from build123d import *

# Parameters (mm, degrees)
SKETCH1_W               = 60
SKETCH1_H               = 160
BOSS_EXTRUDE1_DEPTH     = 3.175
M4_5_THROUGH_DEPTH      = 6.35
M4_5_THROUGH_DEPTH_BACK = 3.175
SKETCH3_R               = 2.75
SKETCH3_R_2             = 2.25
SKETCH4_R               = 1.5
M3_DRILL_DEPTH          = 8
SKETCH5_R               = 2.25
M4_THROUGH_DEPTH        = 6.35
SKETCH6_R               = 2.5
M5_DRILL_DEPTH          = 6.35
SKETCH7_R               = 2.75
M5_THROUGH_DEPTH        = 6.35
SKETCH8_W               = 60
SKETCH8_H               = 30.2375
CUT_EXTRUDE3_DEPTH      = 6.35


with BuildPart() as part:
    # Sketch1 → Boss-Extrude1 (new, symmetric)
    with BuildSketch(Plane(origin=(0, 0, 0), x_dir=(1, 0, 0), z_dir=(0, 1, 0))):
        Rectangle(SKETCH1_W, SKETCH1_H)
    extrude(amount=BOSS_EXTRUDE1_DEPTH, both=True)

    # Sketch3 → M4/5_through (cut, two sides: drawn at the far end of the back side and taken through both)
    with BuildSketch(Plane(origin=(0, 0, 0), x_dir=(1, 0, 0), z_dir=(0, 1, 0)).offset(-M4_5_THROUGH_DEPTH_BACK)):
        with Locations(Location((20, 75.2375, 0), (0, 0, 270))):
            Circle(SKETCH3_R)
        with Locations(Location((20, 50.2375, 0), (0, 0, 270))):
            Circle(SKETCH3_R_2)
        with Locations(Location((-20, 50.2375, 0), (0, 0, 270))):
            Circle(SKETCH3_R_2)
        with Locations(Location((-20, 75.2375, 0), (0, 0, 270))):
            Circle(SKETCH3_R)
        with Locations(Location((0, 75.2375, 0), (0, 0, 270))):
            Circle(SKETCH3_R)
        with Locations(Location((0, 50.2375, 0), (0, 0, 270))):
            Circle(SKETCH3_R_2)
        with Locations(Location((20, -44.7625, 0), (0, 0, 270))):
            Circle(SKETCH3_R_2)
        with Locations(Location((-20, -44.7625, 0), (0, 0, 270))):
            Circle(SKETCH3_R_2)
        with Locations(Location((0, -44.7625, 0), (0, 0, 270))):
            Circle(SKETCH3_R_2)
    extrude(amount=M4_5_THROUGH_DEPTH + M4_5_THROUGH_DEPTH_BACK, mode=Mode.SUBTRACT)

    # Sketch4 → M3_DRILL (cut)
    with BuildSketch(Plane(origin=(0, 0, -80), x_dir=(-1, 0, 0), z_dir=(0, 0, -1))):
        with Locations((-12, 0)):
            Circle(SKETCH4_R)
        with Locations(Location((12, 0, 0), (0, 0, 180))):
            Circle(SKETCH4_R)
    extrude(amount=-M3_DRILL_DEPTH, mode=Mode.SUBTRACT)

    # Sketch5 → M4_through (cut)
    with BuildSketch(Plane(origin=(0, 3.175, 0), x_dir=(1, 0, 0), z_dir=(0, 1, 0))):
        with Locations(Location((-25.2375, -27.6625, 0), (0, 0, 270))):
            Circle(SKETCH5_R)
        with Locations(Location((25.2375, -27.6625, 0), (0, 0, 270))):
            Circle(SKETCH5_R)
        with Locations(Location((25.2375, 33.1375, 0), (0, 0, 270))):
            Circle(SKETCH5_R)
        with Locations(Location((-25.2375, 33.1375, 0), (0, 0, 270))):
            Circle(SKETCH5_R)
    extrude(amount=-M4_THROUGH_DEPTH, mode=Mode.SUBTRACT)

    # Sketch6 → M5_DRILL (cut)
    with BuildSketch(Plane(origin=(0, 3.175, 0), x_dir=(1, 0, 0), z_dir=(0, 1, 0))):
        with Locations(Location((0, 30, 0), (0, 0, 270))):
            Circle(SKETCH6_R)
        with Locations(Location((9.53, 30, 0), (0, 0, 270))):
            Circle(SKETCH6_R)
        with Locations(Location((-9.53, 30, 0), (0, 0, 270))):
            Circle(SKETCH6_R)
    extrude(amount=-M5_DRILL_DEPTH, mode=Mode.SUBTRACT)

    # Sketch7 → M5_through (cut)
    with BuildSketch(Plane(origin=(0, 3.175, 0), x_dir=(1, 0, 0), z_dir=(0, 1, 0))):
        with Locations(Location((0, 10, 0), (0, 0, 270))):
            Circle(SKETCH7_R)
        with Locations(Location((0, -15, 0), (0, 0, 270))):
            Circle(SKETCH7_R)
        with Locations(Location((9.53, 10, 0), (0, 0, 270))):
            Circle(SKETCH7_R)
        with Locations(Location((9.53, -15, 0), (0, 0, 270))):
            Circle(SKETCH7_R)
        with Locations(Location((-9.53, 10, 0), (0, 0, 270))):
            Circle(SKETCH7_R)
        with Locations(Location((-9.53, -15, 0), (0, 0, 270))):
            Circle(SKETCH7_R)
    extrude(amount=-M5_THROUGH_DEPTH, mode=Mode.SUBTRACT)

    # Sketch8 → Cut-Extrude3 (cut)
    with BuildSketch(Plane(origin=(0, 3.175, 0), x_dir=(1, 0, 0), z_dir=(0, 1, 0))):
        with Locations((0, -64.88125)):
            Rectangle(SKETCH8_W, SKETCH8_H)
    extrude(amount=-CUT_EXTRUDE3_DEPTH, mode=Mode.SUBTRACT)


solid = part.part
Source: CAD feature listing. Evaluate the final solid. Frame: model axes, mm. A direction names the side the tool comes from. Coordinates: 2 decimals unless noted, no trailing zeros. Loops run counter-clockwise (first coordinate to the right, second up) from the corner with the lowest first, then second, coordinate; pieces in that order, holes last. Notation, with made-up numbers: (-23.75, 24.25) - (-17.75, 24.25) arc R24 ccw to (-17.75, 57.25) - close; hole circle Ø7 at (-34, -12.5). An arc over 180 degrees is marked (long way). One line per item, written item: value. Start each with the question number.
1. Set-up query: faces 4 (the cylindrical face through (0.099, -0.044, 42.515)), 5 (the cylindrical face through (13.5, 0.07, -76.06)). Return all of +Z, -Z, +X, -X, +Y, -Y with unobstructed straight access to the full face (end or side cutting, diameter ignored); none if empty.
2. Ray query, L1, parallel to Z at x = 20, y = -1.25; L2, parallel to Y at x = 12, z = -73.75 (3 decimals); L3, parallel to Z at x = -25, y = -2.5. Return the intervals inside material, ascending.
3. Mould query, pull axis X, two halves, no side actions, for faces 1 (the flat face through (30, 0, -14)), 2 (the cylindrical face through (20.121, -0.044, -77.985)), 3 (the flat face through (0, 3.175, -16)). Classes: pulls with the +X half, pulls with the -X half, needs draft (parallel to the pull), parting line crosses it, or undercut.
4. Section A-A (x = 0). State how many separate pieces and enclosed holes the cut face has, and give its area (3 significant figures).
5. Section B-B (z = 15). Return the cut outline in (x, y) (3 decimals), and give its area (3 significant figures).
6. Section C-C (x = -20). Return the cut outline in (y, z) (1 decimal).
Verdict:
1. face 4: +Y, -Y
1. face 5: -Z
2. L1: z = -80 to -77.99, -72.49 to -52.49, -47.99 to 42.51, 47.01 to 49.76
2. L2: y = -3.175 to -1.5, 1.5 to 3.175
2. L3: z = -80 to -35.37, -30.9 to 25.43, 29.9 to 49.76
3. face 1: pulls with the +X half
3. face 2: undercut
3. face 3: needs draft
4. separate pieces: 7
4. enclosed holes: 0
4. area: 630 mm2
5. outline: (-30, -3.175) - (-12.28, -3.175) - (-12.28, 3.175) - (-30, 3.175) - close; (-6.78, -3.175) - (-2.75, -3.175) - (-2.75, 3.175) - (-6.78, 3.175) - close; (2.75, -3.175) - (6.78, -3.175) - (6.78, 3.175) - (2.75, 3.175) - close; (12.28, -3.175) - (30, -3.175) - (30, 3.175) - (12.28, 3.175) - close
5. area: 276 mm2
6. outline: (-3.2, -80) - (3.2, -80) - (3.2, -78) - (-3.2, -78) - close; (-3.2, -72.5) - (3.2, -72.5) - (3.2, -52.5) - (-3.2, -52.5) - close; (-3.2, -48) - (3.2, -48) - (3.2, 42.5) - (-3.2, 42.5) - close; (-3.2, 47) - (3.2, 47) - (3.2, 49.8) - (-3.2, 49.8) - close
